Verification items for the finished model (mm, model axes). A direction names the side the tool comes from. Give positions to 0.01 mm unless a question says otherwise; leave off trailing zeros. Write each loop counter-clockwise with the first axis right and the second up, starting at its lowest first coordinate (ties: lowest second). Pieces come first, ordered by that corner, then holes. Notation, with made-up numbers: (18.25, 85.25) - (23.25, 85.25) arc R36 ccw to (23.25, 124.25) - close; hole circle Ø3 at (-25.75, -29). An arc over 180 degrees is marked (long way). Answer as a JSON object with one key per item and string values. Group by question number.
Item 1: Go/stop test with flat-tipped pins: pin 1 (6 mm diameter, centred on y = 10.5, z = 9, fed in from -X); pin 2 (5 mm diameter, centred on x = 41, y = 12.5, fed in from +Z); pin 3 (1.5 mm diameter, centred on y = 1.5, z = 36, fed in from -X). Record where each tip stops, or that it passes through.
Item 2: Sectioned sample at A-A, the plane x = 51. Record the boundary of the cut face in (y, z).
Item 3: Sectioned sample at C-C, the plane z = 40. Record the boundary of the cut face in (x, y), and give its area (3 significant figures).
Item 4: Tool access check on faces 1 (the face through (44, 2, 35)), 2 (the face through (7, 10, 13)), 3 (the face through (38.4, 12.1, 39)), 4 (the face through (13, 3, 37)). Record the directions out of +Z, -Z, +X, -X, +Y, -Y that give a thin tool (end or side, any length) a straight path to the whole face; none if there is none.
Item 5: Sectioned sample at D-D, the plane y = 1.5. Record the boundary of the cut face in (x, z).
Item 6: Scan lines: line 1 along Z through (x, y) = (49, 2.5); line 2 along X through (y, z) = (8, 24); line 3 along Z through (x, y) = (31, 12.25). Record each from-to range of solid material in increasing order. Write a range as [from, to].
Item 7: Sectioned sample at B-B, the plane x = 28. Record the boundary of the cut face in (y, z), and give its area (3 significant figures).
Autodesk Fusion 360 part; units mm, degrees
sketch "Sketch1" plane through (0, 0, 0) normal (0, 1, 0) x (1, 0, 0)
  line L0 (0, 0) -> (53, 0)
  line L1 (53, 0) -> (53, -39)
  line L2 (53, -39) -> (0, -39)
  line L3 (0, -39) -> (0, 0)
  dimension "d1" = 53
  dimension "d2" = 39
extrude "Extrude1" add sketch "Sketch1" along normal blind 20
sketch "Sketch2" plane through (0, 0, 39) normal (0, 0, 1) x (-1, 0, 0)
  line L0 (0, 0) -> (-53, 0)
  line L1 (-53, 0) -> (-53, -20)
  line L2 (-53, -20) -> (0, -20)
  line L3 (0, -20) -> (0, 0)
  line L4 (0, -20) -> (-7, -20)
  line L5 (-7, -20) -> (-7, 0)
  line L6 (-7, 0) -> (0, 0)
  line L7 (0, 0) -> (0, -20)
  line L8 (-53, -20) -> (-46, -20)
  line L9 (-46, -20) -> (-46, 0)
  line L10 (-46, 0) -> (-53, 0)
  line L11 (-53, 0) -> (-53, -20)
  dimension "d5" = 7
  dimension "d6" = 7
extrude "Extrude2" cut sketch "Sketch2" against normal blind 10 contours L0 L2 L3 L4 L5 L6 L7 | L0 L1 L2 L8 L9 L10 L11
sketch "Sketch3" plane through (0, 0, 0) normal (0, 0, -1) x (1, 0, 0)
  line L0 (53, 0) -> (0, 0)
  line L1 (0, 0) -> (0, -20)
  line L2 (0, -20) -> (53, -20)
  line L3 (53, -20) -> (53, 0)
  line L4 (0, 0) -> (7, 0)
  line L5 (7, 0) -> (7, -20)
  line L6 (7, -20) -> (0, -20)
  line L7 (0, -20) -> (0, 0)
  line L8 (53, 0) -> (46, 0)
  line L9 (46, 0) -> (46, -20)
  line L10 (46, -20) -> (53, -20)
  line L11 (53, -20) -> (53, 0)
  dimension "d9" = 7
  dimension "d10" = 7
extrude "Extrude3" cut sketch "Sketch3" against normal blind 26 contours L0 L2 L3 L8 L9 L10 L11 | L0 L1 L2 L4 L5 L6 L7
sketch "Sketch4" plane through (0, 0, 39) normal (0, 0, 1) x (-1, 0, 0)
  line L0 (-7, -20) -> (-7, 0)
  line L1 (-7, 0) -> (-46, 0)
  line L2 (-46, 0) -> (-46, -20)
  line L3 (-46, -20) -> (-7, -20)
  line L4 (-7, -20) -> (-13, -20)
  line L5 (-13, -20) -> (-13, 0)
  line L6 (-13, 0) -> (-7, 0)
  line L7 (-7, 0) -> (-7, -20)
  circle A0 centre (-36, -10) radius 10
  circle A1 centre (-36, -10) radius 6.5
  circle A2 centre (-36, -10) radius 3
  spline S0 degree 5 poles (-13, -15.0203) (-12.838, -14.8194) (-12.5281, -14.4176) (-12.1057, -13.8151) (-11.6287, -13.012) (-11.1861, -12.0086) (-10.9107, -11.0057) (-10.8163, -10.0034) (-10.9104, -9.0017) (-11.1856, -8.0005) (-11.6282, -6.9998) (-12.1053, -6.1997) (-12.5279, -5.5998) (-12.8379, -5.1999) (-13, -5) knots 0 0 0 0 0 0 0.1 0.2 0.3 0.4 0.5 0.6 0.7 0.8 0.9 1 1 1 1 1 1
  point P0 (-13, -10)
  point P1 (-13, -15.0203)
  point P2 (-13, -5)
  point P3 (-10.8633, -10)
  dimension "d13" = 6
  dimension "d14" = 20
  dimension "d15" = 13
  dimension "d16" = 6
extrude "Extrude4" cut sketch "Sketch4" against normal blind 4 contours L0 L1 L3 L4 L5 L6 L7 S0 | L2 L3 A0 | L1 L2 A0
extrude "Extrude5" cut sketch "Sketch4" against normal blind 1 contours L1 L3 L5 A0 | L2 L3 A0 | L5 S0 | L1 L2 A0
extrude "Extrude6" add sketch "Sketch4" along normal blind 5 contours A2
sketch "Sketch5" plane through (0, 0, 29) normal (0, 0, 1) x (-1, 0, 0)
  line L0 (-53, 0) -> (-53, -20)
  line L1 (-53, -20) -> (-46, -20)
  line L2 (-46, -20) -> (-46, 0)
  line L3 (-46, 0) -> (-53, 0)
  line L4 (-53, 0) -> (-51, 0)
  line L5 (-51, 0) -> (-51, -5)
  line L6 (-51, -5) -> (-53, -5)
  line L7 (-53, -5) -> (-53, 0)
  circle A0 centre (-51, -5) radius 2
  line L8 (-53, -20) -> (-51, -20)
  line L9 (-51, -20) -> (-51, -15)
  line L10 (-51, -15) -> (-53, -15)
  line L11 (-53, -15) -> (-53, -20)
  circle A1 centre (-51, -15) radius 2
  dimension "d23" = 2
  dimension "d24" = 5
  dimension "d25" = 4
  dimension "d26" = 2
  dimension "d27" = 5
  dimension "d28" = 4
extrude "Extrude7" cut sketch "Sketch5" against normal blind 3 contours L5 L6 A0 | L5 L6 A0 | L9 L10 A1 | L9 L10 A1
ref_plane "WorkPlane1" through (26.5, 0, 0) normal (1, 0, 0) x (0, 1, 0)
mirror "Mirror1" about plane through (26.5, 0, 0) normal (1, 0, 0) of "Extrude7"
Geometry check:
{
 "1": {"pin 1": "x = 7", "pin 2": "z = 39", "pin 3": "x = 13"},
 "2": {"outline": "(0, 26) - (3, 26) - (3, 29) - (0, 29) - close; (7, 26) - (13, 26) - (13, 29) - (7, 29) - close; (17, 26) - (20, 26) - (20, 29) - (17, 29) - close"},
 "3": {"outline": "circle Ø6 at (36, 10)", "area": "28.3 mm^2"},
 "4": {"face 1": "+Z, +X, -Y", "face 2": "-Z, -X, +Y, -Y", "face 3": "+Z", "face 4": "+Z, -X, -Y"},
 "5": {"outline": "(0, 26) - (7, 26) - (7, 0) - (46, 0) - (46, 26) - (53, 26) - (53, 29) - (46, 29) - (46, 35) - (41.27, 35) - (41.27, 39) - (30.73, 39) - (30.73, 38) - (13, 38) - (13, 35) - (7, 35) - (7, 29) - (0, 29) - close"},
 "6": {"line 1": "[26, 29]", "line 2": "[7, 46]", "line 3": "[0, 39]"},
 "7": {"outline": "(0, 0) - (20, 0) - (20, 38) - (16, 38) - (16, 39) - (4, 39) - (4, 38) - (0, 38) - close", "area": "772 mm^2"}
}
